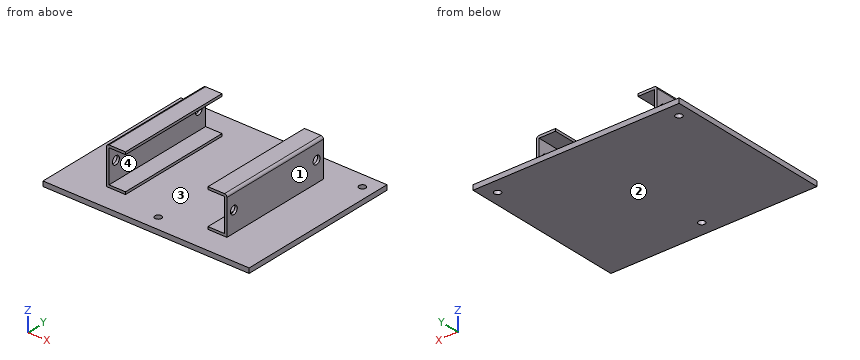
from build123d import *

# Parameters (mm, degrees)
F0_W     = 125
F0_H     = 100
F0_R     = 2
F1_DEPTH = 3
F4_DEPTH = 70
F5_R     = 2.5
F6_DEPTH = 99.001
F7_R     = 1.5


with BuildPart() as f1:
    # F0 (on Top) → F1 (new body)
    with BuildSketch(Plane.XY):
        Rectangle(F0_W, F0_H)
        with Locations((0, -41.15)):
            Circle(F0_R, mode=Mode.SUBTRACT)
        with Locations((-55, 41.15)):
            Circle(F0_R, mode=Mode.SUBTRACT)
        with Locations((55, 41.15)):
            Circle(F0_R, mode=Mode.SUBTRACT)
    extrude(amount=F1_DEPTH)

    # F3 (on offset) → F4 (join)
    with BuildSketch(Plane.XZ.offset(35)):
        Polygon((35, 24.5), (35, 4.5), (25, 4.5), (25, 3), (36.5, 3), (36.5, 26), (25, 26), (25, 24.5), align=None)
        Polygon((-36.5, 26), (-36.5, 3), (-25, 3), (-25, 4.5), (-35, 4.5), (-35, 24.5), (-25, 24.5), (-25, 26), align=None)
    extrude(amount=-F4_DEPTH)

    # F5 (on face) → F6 (cut, through all)
    with BuildSketch(Plane.YZ.offset(36.5)):
        with Locations((-30, 15.5)):
            Circle(F5_R)
        with Locations((30, 15.5)):
            Circle(F5_R)
    extrude(amount=-F6_DEPTH, mode=Mode.SUBTRACT)

    # F7
    f7_edges = [f1.edges().sort_by_distance(p)[0] for p in [
        (36.5, 0, 26),
        (-36.5, 0, 26),
    ]]
    fillet(f7_edges, radius=F7_R)


solid = f1.part
Work out the finished part from the listing and answer in its coordinate system (mm). Face numbers are marked on the shaded views. Round coordinates to 2 decimals unless told otherwise and drop trailing zeros. Order: outer loops, then holes, each group sorted by start corner. A loop starts at its lowest first (then second) coordinate and runs counter-clockwise, first axis right, second up. Notation, with made-up numbers: M -31,65 L 10,65 A24 cw 10,95 Z; hole C 72.25,9.25 d5. An arc over 180 degrees is marked long. Put each result on its own line as item: value. Start each with the question number.
Q1. Section D-D, the plane y = -41.15 is taken. Write down the section's boundary in (x, z).
Q2. Section B-B, the plane y = 41.15 is taken. Write down the section's boundary in (x, z).
Q3. For a pull along X with two mould halves and no side action, classify the marked faces 1, 2, 3 and 4 as pulls with the +X half, pulls with the -X half, needs draft (parallel to the pull), parting line crosses it, or undercut.
Q4. Flat-ended cylindrical pins translate along their axes: pin 1 (6 mm diameter, centred on x = -32.5, z = 17.5, fed in from -Y); pin 2 (8 mm diameter, centred on y = 37, z = 23.5, fed in from +X); pin 3 (12.5 mm diameter, centred on x = -31.5, z = 14, fed in from +Y); pin 4 (3 mm diameter, centred on y = -30, z = 15.5, fed in from -X). Find the tip coordinate at first contact, or state that the pin passes through.
Q5. Section C-C, the plane z = 15.5 is taken. Write down the section's boundary in (x, y).
Q6. Straight lines are drawn through the part: L1, parallel to X at y = -1.5, z = 16.75; L2, parallel to Z at x = -32, y = 0; L3, parallel to Y at x = 55, z = 1.8. For each, find the intervals that lie inside material, in ascending order. Write a range as [from, to].
Q7. Section A-A, the plane x = 0 is taken. Write down the section's boundary in (y, z), and give its area (3 significant figures).
Findings below:
1. outline: M -62.5,0 L -2,0 L -2,3 L -62.5,3 Z; M 2,0 L 62.5,0 L 62.5,3 L 2,3 Z
2. outline: M -62.5,0 L -57,0 L -57,3 L -62.5,3 Z; M -53,0 L 53,0 L 53,3 L -53,3 Z; M 57,0 L 62.5,0 L 62.5,3 L 57,3 Z
3. face 1: pulls with the +X half
3. face 2: needs draft
3. face 3: undercut
3. face 4: undercut
4. pin 1: stops at y = -35
4. pin 2: stops at x = 36.5
4. pin 3: stops at y = 35
4. pin 4: passes through
5. outline: M -36.5,-35 L -35,-35 L -35,-32.5 L -36.5,-32.5 Z; M -36.5,-27.5 L -35,-27.5 L -35,27.5 L -36.5,27.5 Z; M -36.5,32.5 L -35,32.5 L -35,35 L -36.5,35 Z; M 35,-35 L 36.5,-35 L 36.5,-32.5 L 35,-32.5 Z; M 35,-27.5 L 36.5,-27.5 L 36.5,27.5 L 35,27.5 Z; M 35,32.5 L 36.5,32.5 L 36.5,35 L 35,35 Z
6. L1: x = [-36.5, -35], [35, 36.5]
6. L2: z = [0, 4.5], [24.5, 26]
6. L3: y = [-50, 39.15], [43.15, 50]
7. outline: M -50,0 L -43.15,0 L -43.15,3 L -50,3 Z; M -39.15,0 L 50,0 L 50,3 L -39.15,3 Z
7. area: 288 mm^2
